Check sheet for the modelled part. Datum: model origin and axes. Units: mm. A direction names the side the tool comes from. Coordinates: 2 decimals unless noted, no trailing zeros. Loops run counter-clockwise (first coordinate to the right, second up) from the corner with the lowest first, then second, coordinate; pieces in that order, holes last.
```python
from build123d import *

# Parameters (mm, degrees)
SKETCH1_R           = 10
BOSS_EXTRUDE1_DEPTH = 10
SKETCH2_R           = 20
BOSS_EXTRUDE2_DEPTH = 2
BOSS_EXTRUDE3_START = -2
SKETCH3_R           = 20
BOSS_EXTRUDE3_DEPTH = 2
BOSS_EXTRUDE4_START = 18.5
SKETCH4_R           = 10
SKETCH4_R_2         = 0.05
BOSS_EXTRUDE4_DEPTH = 18.5
SKETCH5_R           = 11
BOSS_EXTRUDE5_DEPTH = 3.5


with BuildPart() as part:
    # Sketch1 → Boss-Extrude1 (new body)
    with BuildSketch(Plane.XY):
        with BuildLine():
            Line((0, 17), (1.023829773, 13.962513119))
            ThreePointArc((1.023829773, 13.962513119), (1.372239965, 13.932586173), (1.719794009, 13.893966625))
            Line((1.719794009, 13.893966625), (3.316535474, 16.673349767))
            Line((3.316535474, 16.673349767), (3.728108352, 13.494488064))
            ThreePointArc((3.728108352, 13.494488064), (4.063985482, 13.3971647), (4.397327072, 13.291482785))
            Line((4.397327072, 13.291482785), (6.50561835, 15.705952053))
            Line((6.50561835, 15.705952053), (6.289117817, 12.507877401))
            ThreePointArc((6.289117817, 12.507877401), (6.599554316, 12.346897701), (6.905873322, 12.178214715))
            Line((6.905873322, 12.178214715), (9.444693961, 14.134983409))
            Line((9.444693961, 14.134983409), (8.608440012, 11.040596024))
            ThreePointArc((8.608440012, 11.040596024), (8.881505978, 10.822146347), (9.149030733, 10.596944684))
            Line((9.149030733, 10.596944684), (12.02081528, 12.02081528))
            Line((12.02081528, 12.02081528), (10.596944684, 9.149030733))
            ThreePointArc((10.596944684, 9.149030733), (10.822146347, 8.881505978), (11.040596024, 8.608440012))
            Line((11.040596024, 8.608440012), (14.134983409, 9.444693961))
            Line((14.134983409, 9.444693961), (12.178214715, 6.905873322))
            ThreePointArc((12.178214715, 6.905873322), (12.346897701, 6.599554316), (12.507877401, 6.289117817))
            Line((12.507877401, 6.289117817), (15.705952053, 6.50561835))
            Line((15.705952053, 6.50561835), (13.291482785, 4.397327072))
            ThreePointArc((13.291482785, 4.397327072), (13.3971647, 4.063985482), (13.494488064, 3.728108352))
            Line((13.494488064, 3.728108352), (16.673349767, 3.316535474))
            Line((16.673349767, 3.316535474), (13.893966625, 1.719794009))
            ThreePointArc((13.893966625, 1.719794009), (13.932586173, 1.372239965), (13.962513119, 1.023829773))
            Line((13.962513119, 1.023829773), (17, 0))
            Line((17, 0), (13.962513119, -1.023829773))
            ThreePointArc((13.962513119, -1.023829773), (13.932586173, -1.372239965), (13.893966625, -1.719794009))
            Line((13.893966625, -1.719794009), (16.673349767, -3.316535474))
            Line((16.673349767, -3.316535474), (13.494488064, -3.728108352))
            ThreePointArc((13.494488064, -3.728108352), (13.3971647, -4.063985482), (13.291482785, -4.397327072))
            Line((13.291482785, -4.397327072), (15.705952053, -6.50561835))
            Line((15.705952053, -6.50561835), (12.507877401, -6.289117817))
            ThreePointArc((12.507877401, -6.289117817), (12.346897701, -6.599554316), (12.178214715, -6.905873322))
            Line((12.178214715, -6.905873322), (14.134983409, -9.444693961))
            Line((14.134983409, -9.444693961), (11.040596024, -8.608440012))
            ThreePointArc((11.040596024, -8.608440012), (10.822146347, -8.881505978), (10.596944684, -9.149030733))
            Line((10.596944684, -9.149030733), (12.02081528, -12.02081528))
            Line((12.02081528, -12.02081528), (9.149030733, -10.596944684))
            ThreePointArc((9.149030733, -10.596944684), (8.881505978, -10.822146347), (8.608440012, -11.040596024))
            Line((8.608440012, -11.040596024), (9.444693961, -14.134983409))
            Line((9.444693961, -14.134983409), (6.905873322, -12.178214715))
            ThreePointArc((6.905873322, -12.178214715), (6.599554316, -12.346897701), (6.289117817, -12.507877401))
            Line((6.289117817, -12.507877401), (6.50561835, -15.705952053))
            Line((6.50561835, -15.705952053), (4.397327072, -13.291482785))
            ThreePointArc((4.397327072, -13.291482785), (4.063985482, -13.3971647), (3.728108352, -13.494488064))
            Line((3.728108352, -13.494488064), (3.316535474, -16.673349767))
            Line((3.316535474, -16.673349767), (1.719794009, -13.893966625))
            ThreePointArc((1.719794009, -13.893966625), (1.372239965, -13.932586173), (1.023829773, -13.962513119))
            Line((1.023829773, -13.962513119), (0, -17))
            Line((0, -17), (-1.023829773, -13.962513119))
            ThreePointArc((-1.023829773, -13.962513119), (-1.372239965, -13.932586173), (-1.719794009, -13.893966625))
            Line((-1.719794009, -13.893966625), (-3.316535474, -16.673349767))
            Line((-3.316535474, -16.673349767), (-3.728108352, -13.494488064))
            ThreePointArc((-3.728108352, -13.494488064), (-4.063985482, -13.3971647), (-4.397327072, -13.291482785))
            Line((-4.397327072, -13.291482785), (-6.50561835, -15.705952053))
            Line((-6.50561835, -15.705952053), (-6.289117817, -12.507877401))
            ThreePointArc((-6.289117817, -12.507877401), (-6.599554316, -12.346897701), (-6.905873322, -12.178214715))
            Line((-6.905873322, -12.178214715), (-9.444693961, -14.134983409))
            Line((-9.444693961, -14.134983409), (-8.608440012, -11.040596024))
            ThreePointArc((-8.608440012, -11.040596024), (-8.881505978, -10.822146347), (-9.149030733, -10.596944684))
            Line((-9.149030733, -10.596944684), (-12.02081528, -12.02081528))
            Line((-12.02081528, -12.02081528), (-10.596944684, -9.149030733))
            ThreePointArc((-10.596944684, -9.149030733), (-10.822146347, -8.881505978), (-11.040596024, -8.608440012))
            Line((-11.040596024, -8.608440012), (-14.134983409, -9.444693961))
            Line((-14.134983409, -9.444693961), (-12.178214715, -6.905873322))
            ThreePointArc((-12.178214715, -6.905873322), (-12.346897701, -6.599554316), (-12.507877401, -6.289117817))
            Line((-12.507877401, -6.289117817), (-15.705952053, -6.50561835))
            Line((-15.705952053, -6.50561835), (-13.291482785, -4.397327072))
            ThreePointArc((-13.291482785, -4.397327072), (-13.3971647, -4.063985482), (-13.494488064, -3.728108352))
            Line((-13.494488064, -3.728108352), (-16.673349767, -3.316535474))
            Line((-16.673349767, -3.316535474), (-13.893966625, -1.719794009))
            ThreePointArc((-13.893966625, -1.719794009), (-13.932586173, -1.372239965), (-13.962513119, -1.023829773))
            Line((-13.962513119, -1.023829773), (-17, 0))
            Line((-17, 0), (-13.962513119, 1.023829773))
            ThreePointArc((-13.962513119, 1.023829773), (-13.932586173, 1.372239965), (-13.893966625, 1.719794009))
            Line((-13.893966625, 1.719794009), (-16.673349767, 3.316535474))
            Line((-16.673349767, 3.316535474), (-13.494488064, 3.728108352))
            ThreePointArc((-13.494488064, 3.728108352), (-13.3971647, 4.063985482), (-13.291482785, 4.397327072))
            Line((-13.291482785, 4.397327072), (-15.705952053, 6.50561835))
            Line((-15.705952053, 6.50561835), (-12.507877401, 6.289117817))
            ThreePointArc((-12.507877401, 6.289117817), (-12.346897701, 6.599554316), (-12.178214715, 6.905873322))
            Line((-12.178214715, 6.905873322), (-14.134983409, 9.444693961))
            Line((-14.134983409, 9.444693961), (-11.040596024, 8.608440012))
            ThreePointArc((-11.040596024, 8.608440012), (-10.822146347, 8.881505978), (-10.596944684, 9.149030733))
            Line((-10.596944684, 9.149030733), (-12.02081528, 12.02081528))
            Line((-12.02081528, 12.02081528), (-9.149030733, 10.596944684))
            ThreePointArc((-9.149030733, 10.596944684), (-8.881505978, 10.822146347), (-8.608440012, 11.040596024))
            Line((-8.608440012, 11.040596024), (-9.444693961, 14.134983409))
            Line((-9.444693961, 14.134983409), (-6.905873322, 12.178214715))
            ThreePointArc((-6.905873322, 12.178214715), (-6.599554316, 12.346897701), (-6.289117817, 12.507877401))
            Line((-6.289117817, 12.507877401), (-6.50561835, 15.705952053))
            Line((-6.50561835, 15.705952053), (-4.397327072, 13.291482785))
            ThreePointArc((-4.397327072, 13.291482785), (-4.063985482, 13.3971647), (-3.728108352, 13.494488064))
            Line((-3.728108352, 13.494488064), (-3.316535474, 16.673349767))
            Line((-3.316535474, 16.673349767), (-1.719794009, 13.893966625))
            ThreePointArc((-1.719794009, 13.893966625), (-1.372239965, 13.932586173), (-1.023829773, 13.962513119))
            Line((-1.023829773, 13.962513119), (0, 17))
        make_face()
        Circle(SKETCH1_R, mode=Mode.SUBTRACT)
    extrude(amount=BOSS_EXTRUDE1_DEPTH)

    # Sketch2 → Boss-Extrude2 (add)
    with BuildSketch(Plane.XY.offset(10)):
        Circle(SKETCH2_R)
    extrude(amount=-BOSS_EXTRUDE2_DEPTH)

    # Sketch3 → Boss-Extrude3 (add)
    with BuildSketch(Plane(origin=(0, 0, 0), x_dir=(-1, 0, 0), z_dir=(0, 0, -1)).offset(BOSS_EXTRUDE3_START)):
        with Locations(Location((0, 0, 0), (0, 0, 180))):
            Circle(SKETCH3_R)
    extrude(amount=BOSS_EXTRUDE3_DEPTH)

    # Sketch4 → Boss-Extrude4 (add)
    with BuildSketch(Plane(origin=(0, 0, 0), x_dir=(-1, 0, 0), z_dir=(0, 0, -1)).offset(BOSS_EXTRUDE4_START)):
        Circle(SKETCH4_R)
        Circle(SKETCH4_R_2, mode=Mode.SUBTRACT)
    extrude(amount=-BOSS_EXTRUDE4_DEPTH)

    # Sketch5 → Boss-Extrude5 (add)
    with BuildSketch(Plane(origin=(0, 0, 0), x_dir=(-1, 0, 0), z_dir=(0, 0, -1))):
        with Locations(Location((0, 0, 0), (0, 0, 180))):
            Circle(SKETCH5_R)
    extrude(amount=BOSS_EXTRUDE5_DEPTH)


solid = part.part
```
1) Section check C-C on x = 15. Enter the section's corners in (y, z).
Answer sheet:
outline: (-13.23, 0) - (13.23, 0) - (13.23, 2) - (6.46, 2) - (6.46, 8) - (13.23, 8) - (13.23, 10) - (-13.23, 10) - (-13.23, 8) - (-6.46, 8) - (-6.46, 2) - (-13.23, 2) - close; hole (-5.89, 2) - (-3.53, 2) - (-3.53, 8) - (-5.89, 8) - close; hole (-2.36, 2) - (-0.67, 2) - (-0.67, 8) - (-2.36, 8) - close; hole (0.67, 2) - (2.36, 2) - (2.36, 8) - (0.67, 8) - close; hole (3.53, 2) - (5.89, 2) - (5.89, 8) - (3.53, 8) - close
2) Section check B-B on z = -8.25. Enter the section's corners in (x, y), plus the area to 3 significant figures.
Answer sheet:
outline: circle Ø20 at (0, 0); hole circle Ø0.1 at (0, 0)
area: 314 mm2
3) Mould release check, pull along Z, two halves, no side actions. Record for faces 4 (the flat face through (9, 9, 0)), 5 (the flat face through (8.19, -13.17, 4.96)), 6 (the flat face through (0, 0, 10)): +Z half, -Z half, draft (parallel to the pull), parting line (faces both ways), or undercut.
Answer sheet:
face 4: -Z half
face 5: undercut
face 6: +Z half
4) Section check A-A on x = 5. Enter the section's corners in (y, z).
Answer sheet:
outline: (-19.36, 0) - (-9.8, 0) - (-9.8, -3.5) - (-8.66, -3.5) - (-8.66, -18.5) - (8.66, -18.5) - (8.66, -3.5) - (9.8, -3.5) - (9.8, 0) - (19.36, 0) - (19.36, 2) - (13.98, 2) - (13.98, 8) - (19.36, 8) - (19.36, 10) - (-19.36, 10) - (-19.36, 8) - (-13.98, 8) - (-13.98, 2) - (-19.36, 2) - close; hole (-8.66, 2) - (8.66, 2) - (8.66, 8) - (-8.66, 8) - close
5) Depth check by flat-ended pin: pin 1 (2 mm diameter, centred on y = -4, z = -8, fed in from -X); pin 2 (3 mm diameter, centred on x = 10.5, z = 2.5, fed in from +Y); pin 3 (2 mm diameter, centred on x = 3, y = -11, fed in from -Z). Enter the tip coordinate at first touch or a pass-through.
Answer sheet:
pin 1: stops at x = -9.54
pin 2: stops at y = 17.82
pin 3: stops at z = -3.5
6) Scan lines: line 1 (Z direction, x = 13, y = 10.5); line 2 (Z direction, x = 8.5, y = -3.5); line 3 (Z direction, x = -15, y = -3). Record each from-to range of solid material in increasing order.
Answer sheet:
line 1: z = 0 to 2, 8 to 10
line 2: z = -18.5 to 2, 8 to 10
line 3: z = 0 to 10
7) Set-up check for faces 1 (the flat face through (-0.505, -15.503, 4.958)), 2 (the flat face through (-5.47, 14.52, 4.96)), 3 (the flat face through (-12.57, -9.02, 4.96)): record each of +Z, -Z, +X, -X, +Y, -Y from which the full face is reachable in a straight line by a thin tool's end or side.
Answer sheet:
face 1: -Y
face 2: +Y
face 3: none
